For this review, use the dimensioned drawing (mm, ordinates from the lowest corner) and the shaded views. A direction names the side the tool comes from. Give positions to 0.01 mm unless a question says otherwise; leave off trailing zeros. Loops run counter-clockwise (first coordinate to the right, second up) from the corner with the lowest first, then second, coordinate; pieces in that order, holes last. Notation, with made-up numbers: (53, -12.5) -> (101, -12.5) arc R18 cw to (101, 10.5) -> close; hole circle Ø1 at (-4, 61). An arc over 180 degrees is marked (long way). Use a Markdown table: item, result. Add a question column.
1. Add section A-A (x = 4). State the section outline as (y, z) points, and give its area (3 significant figures).
2. For pin 1 Ø1.5 at (y, z) = (28.5, 17) entering from +X; pin 2 Ø1.5 at (x, z) = (11.5, 13.5) entering from +Y; pin 3 Ø5 at (x, z) = (11, 18) entering from -Y, all flat-tipped, find the tip position at first contact; note any pin that passes through.
3. Add section C-C (y = 15.5). State the section outline as (x, z) points.
4. Add section B-B (z = 16). State the section outline as (x, y) points (1 decimal), and give its area (3 significant figures).
5. To check wall thickness, follow line 1 (X direction, y = 26, z = 17); line 2 (Z direction, x = 2.5, y = 47.5); line 3 (Y direction, x = 12, z = 13.5). State the ranges of each line that lie inside material, in increasing order.
6. For the marked faces 1, 2 and 3, list the 3-axis set-ups (+Z, -Z, +X, -X, +Y, -Y) from which the entire face can be reached by the end or side of a thin tool; tool diameter is ignored.
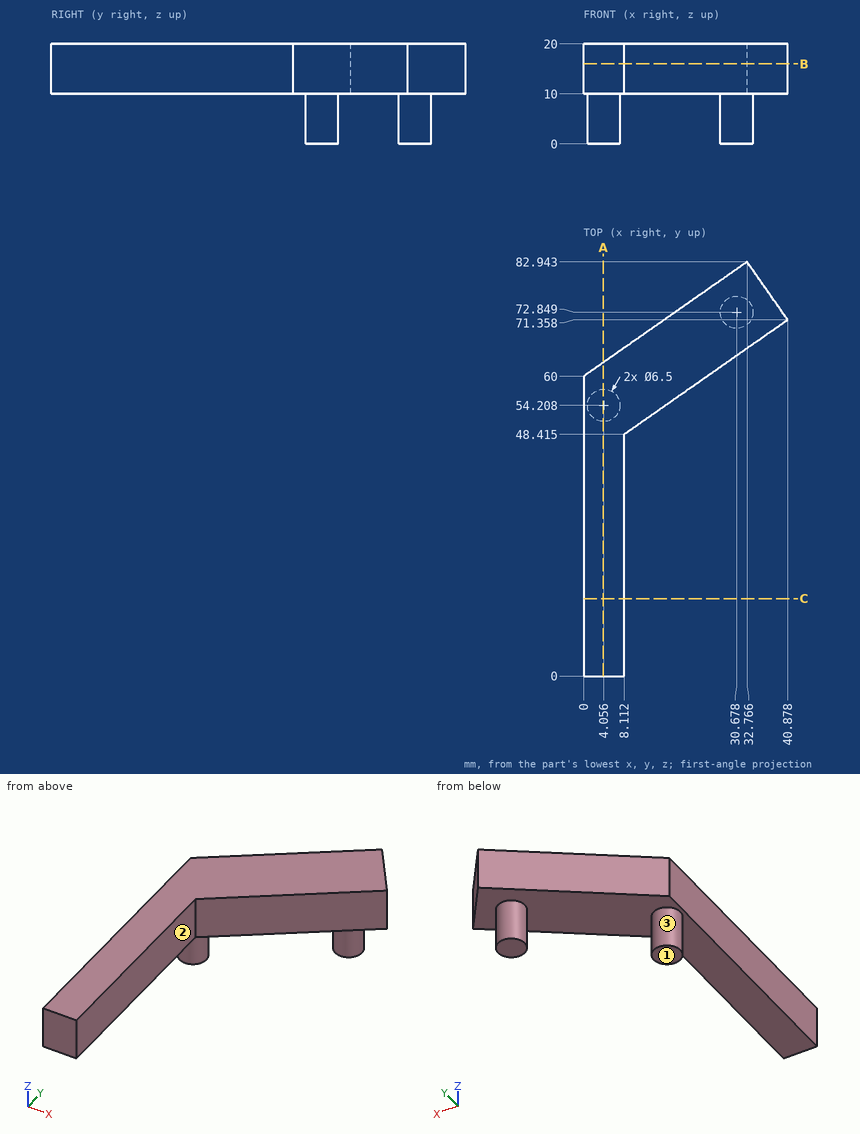
Taken from the geometry:
| question | item | result |
|---|---|---|
| 1 | outline | (0, 10) -> (50.96, 10) -> (50.96, 0) -> (57.46, 0) -> (57.46, 10) -> (62.8, 10) -> (62.8, 20) -> (0, 20) -> close |
| 1 | area | 693 mm^2 |
| 2 | pin 1 | stops at x = 8.11 |
| 2 | pin 2 | stops at y = 68.58 |
| 2 | pin 3 | stops at y = 48.69 |
| 3 | outline | (0, 10) -> (8.11, 10) -> (8.11, 20) -> (0, 20) -> close |
| 4 | outline | (0, 0) -> (8.1, 0) -> (8.1, 48.4) -> (40.9, 71.4) -> (32.8, 82.9) -> (0, 60) -> close |
| 4 | area | 1,010 mm^2 |
| 5 | line 1 | x = 0 to 8.11 |
| 5 | line 2 | z = 10 to 20 |
| 5 | line 3 | y = 51.14 to 68.4 |
| 6 | face 1 | -Z, +X, -X, +Y, -Y |
| 6 | face 2 | +Z, -Z, +X, -Y |
| 6 | face 3 | -Z |
